Part model, mm, in its own coordinate system. A direction names the side the tool comes from. Give positions to 0.01 mm unless a question says otherwise; leave off trailing zeros. Order: outer loops, then holes, each group sorted by start corner. A loop starts at its lowest first (then second) coordinate and runs counter-clockwise, first axis right, second up. Notation, with made-up numbers: M 42,81 L 59,81 A18 ccw 59,113 Z; hole C 31,-32.5 d11. An arc over 180 degrees is marked long. One line per question, with ' | ' between items.
```python
from build123d import *

# Parameters (mm, degrees)
SKETCH1_R           = 10.5
BOSS_EXTRUDE1_DEPTH = 35
SKETCH1_3_R         = 3
SKETCH1_3_R_2       = 1.1
BOSS_EXTRUDE2_DEPTH = 4
SKETCH2_R           = 11.5
SKETCH2_R_2         = 10.5
CUT_EXTRUDE1_DEPTH  = 30
SKETCH2_3_R         = 4
SKETCH2_3_R_2       = 1.6
BOSS_EXTRUDE3_DEPTH = 6
FILLET1_R           = 3
SKETCH3_R           = 3
CUT_EXTRUDE2_DEPTH  = 54.516726423


with BuildPart() as part:
    # Sketch1 → Boss-Extrude1 (new body)
    with BuildSketch(Plane.XY):
        with BuildLine():
            ThreePointArc((3, 15), (0, 12), (-3, 15))
            Line((-3, 15), (-3, 19.773719933))
            ThreePointArc((-3, 19.773719933), (-17.320508076, 10), (-18.62454379, -7.288783755))
            Line((-18.62454379, -7.288783755), (-14.490381057, -4.901923789))
            ThreePointArc((-14.490381057, -4.901923789), (-11.490381057, -4.901923789), (-9.990381057, -7.5))
            ThreePointArc((-9.990381057, -7.5), (-10.392304845, -9), (-11.490381057, -10.098076211))
            Line((-11.490381057, -10.098076211), (-15.62454379, -12.484936178))
            ThreePointArc((-15.62454379, -12.484936178), (0, -20), (15.62454379, -12.484936178))
            Line((15.62454379, -12.484936178), (11.490381057, -10.098076211))
            ThreePointArc((11.490381057, -10.098076211), (10.392304845, -6), (14.490381057, -4.901923789))
            Line((14.490381057, -4.901923789), (18.62454379, -7.288783755))
            ThreePointArc((18.62454379, -7.288783755), (19.653127942, -3.708714347), (20, 0))
            ThreePointArc((20, 0), (15.165750888, 13.03840481), (3, 19.773719933))
            Line((3, 19.773719933), (3, 15))
        make_face()
        Circle(SKETCH1_R, mode=Mode.SUBTRACT)
    extrude(amount=BOSS_EXTRUDE1_DEPTH)

    # Sketch1_3 → Boss-Extrude2 (add)
    with BuildSketch(Plane.XY):
        with BuildLine():
            ThreePointArc((15.62454379, -12.484936178), (17.320508076, -10), (18.62454379, -7.288783755))
            Line((18.62454379, -7.288783755), (14.490381057, -4.901923789))
            ThreePointArc((14.490381057, -4.901923789), (15.588457268, -6), (15.990381057, -7.5))
            ThreePointArc((15.990381057, -7.5), (14.490381057, -10.098076211), (11.490381057, -10.098076211))
            Line((11.490381057, -10.098076211), (15.62454379, -12.484936178))
        make_face()
        with Locations((12.990381057, -7.5)):
            Circle(SKETCH1_3_R)
        with Locations((12.990381057, -7.5)):
            Circle(SKETCH1_3_R_2, mode=Mode.SUBTRACT)
        with Locations((-12.990381057, -7.5)):
            Circle(SKETCH1_3_R)
        with Locations((-12.990381057, -7.5)):
            Circle(SKETCH1_3_R_2, mode=Mode.SUBTRACT)
        with BuildLine():
            Line((-14.490381057, -4.901923789), (-18.62454379, -7.288783755))
            ThreePointArc((-18.62454379, -7.288783755), (-17.320508076, -10), (-15.62454379, -12.484936178))
            Line((-15.62454379, -12.484936178), (-11.490381057, -10.098076211))
            ThreePointArc((-11.490381057, -10.098076211), (-15.588457268, -9), (-14.490381057, -4.901923789))
        make_face()
        with BuildLine():
            Line((-3, 19.773719933), (-3, 15))
            ThreePointArc((-3, 15), (0, 18), (3, 15))
            Line((3, 15), (3, 19.773719933))
            ThreePointArc((3, 19.773719933), (0, 20), (-3, 19.773719933))
        make_face()
        with Locations((0, 15)):
            Circle(SKETCH1_3_R)
        with Locations((0, 15)):
            Circle(SKETCH1_3_R_2, mode=Mode.SUBTRACT)
    extrude(amount=BOSS_EXTRUDE2_DEPTH)

    # Sketch2 → Cut-Extrude1 (cut)
    with BuildSketch(Plane.XY.offset(35)):
        Circle(SKETCH2_R)
        Circle(SKETCH2_R_2, mode=Mode.SUBTRACT)
    extrude(amount=-CUT_EXTRUDE1_DEPTH, mode=Mode.SUBTRACT)

    # Sketch2_3 → Boss-Extrude3 (add)
    with BuildSketch(Plane.XY.offset(35)):
        with BuildLine():
            ThreePointArc((-19.595917942, -4), (-20, 0), (-19.595917942, 4))
            Line((-19.595917942, 4), (-31.2, 4))
            ThreePointArc((-31.2, 4), (-28.371572875, 2.828427125), (-27.2, 0))
            ThreePointArc((-27.2, 0), (-28.371572875, -2.828427125), (-31.2, -4))
            Line((-31.2, -4), (-19.595917942, -4))
        make_face()
        with Locations((-31.2, 0)):
            Circle(SKETCH2_3_R)
        with Locations((-31.2, 0)):
            Circle(SKETCH2_3_R_2, mode=Mode.SUBTRACT)
        with BuildLine():
            ThreePointArc((31.2, -4), (27.2, 0), (31.2, 4))
            Line((31.2, 4), (19.595917942, 4))
            ThreePointArc((19.595917942, 4), (19.89872306, 2.01017924), (20, 0))
            ThreePointArc((20, 0), (19.89872306, -2.01017924), (19.595917942, -4))
            Line((19.595917942, -4), (31.2, -4))
        make_face()
        with Locations((31.2, 0)):
            Circle(SKETCH2_3_R)
        with Locations((31.2, 0)):
            Circle(SKETCH2_3_R_2, mode=Mode.SUBTRACT)
    extrude(amount=-BOSS_EXTRUDE3_DEPTH)

    # Fillet1
    fillet1_edges = [part.edges().sort_by_distance(p)[0] for p in [
        (-20, 0, 29),
        (19.595917942, -4, 32),
        (19.595917942, 4, 32),
        (20, 0, 29),
        (-19.595917942, 4, 32),
        (-19.595917942, -4, 32),
    ]]
    fillet(fillet1_edges, radius=FILLET1_R)

    # Sketch3 → Cut-Extrude2 (cut, through all)
    with BuildSketch(Plane(origin=(0, 0, 0), x_dir=(1, 0, 0), z_dir=(0, 1, 0))):
        with Locations(Location((0, -13.5, 0), (0, 0, 270))):
            Circle(SKETCH3_R)
    extrude(amount=-CUT_EXTRUDE2_DEPTH, mode=Mode.SUBTRACT)


solid = part.part
```
1. Slice it at A-A on x = 0. Give the cut face in (y, z), then the cut area to 3 significant figures.
Worked out:
outline: M -20,0 L -10.5,0 L -10.5,5 L -11.5,5 L -11.5,10.5 L -20,10.5 Z; M -20,16.5 L -11.5,16.5 L -11.5,35 L -20,35 Z; M 10.5,0 L 13.9,0 L 13.9,4 L 12,4 L 12,35 L 11.5,35 L 11.5,5 L 10.5,5 Z; M 16.1,0 L 20,0 L 20,4 L 16.1,4 Z | area: 297 mm2
2. Slice it at C-C on z = 20. Give the cut face in (x, y), then the cut area to 3 significant figures.
Worked out:
outline: M -18.62,-7.29 L -14.49,-4.9 A3 cw -11.49,-10.1 L -15.62,-12.48 A20 ccw 15.62,-12.48 L 11.49,-10.1 A3 cw 14.49,-4.9 L 18.62,-7.29 A20 ccw 3,19.77 L 3,15 A3 cw -3,15 L -3,19.77 A20 ccw Z; hole C 0,0 d23 | area: 710 mm2
3. Slice it at D-D on z = 27. Give the cut face in (x, y).
Worked out:
outline: M -19.48,-5.24 A3 cw -19.05,-6.09 A20 ccw -18.62,-7.29 L -14.49,-4.9 A3 cw -11.49,-10.1 L -15.62,-12.48 A20 ccw 15.62,-12.48 L 11.49,-10.1 A3 cw 14.49,-4.9 L 18.62,-7.29 A20 ccw 19.05,-6.09 A3 cw 19.48,-5.24 A20.17 ccw 19.48,5.24 A3 cw 19.05,6.09 A20 ccw 3,19.77 L 3,15 A3 cw -3,15 L -3,19.77 A20 ccw -19.05,6.09 A3 cw -19.48,5.24 A20.17 ccw Z; hole C 0,0 d23
4. Drop flat-ended pins along their axis: pin 1 (5 mm diameter, centred on x = -28.5, z = 32.5, fed in from +Y); pin 2 (4 mm diameter, centred on x = -27.5, y = 1.5, fed in from -Z); pin 3 (2.5 mm diameter, centred on x = 14.5, y = -8.5, fed in from +Z). Give the stop position or say it passes through.
Worked out:
pin 1: stops at y = 4 | pin 2: stops at z = 29 | pin 3: stops at z = 4
5. Slice it at B-B on z = 31.5. Give the cut face in (x, y).
Worked out:
outline: M -31.2,-4 L -21.91,-4 A3 cw -19.05,-6.09 A20 ccw -18.62,-7.29 L -14.49,-4.9 A3 cw -11.49,-10.1 L -15.62,-12.48 A20 ccw 15.62,-12.48 L 11.49,-10.1 A3 cw 14.49,-4.9 L 18.62,-7.29 A20 ccw 19.05,-6.09 A3 cw 21.91,-4 L 31.2,-4 A4 ccw 31.2,4 L 21.91,4 A3 cw 19.05,6.09 A20 ccw 3,19.77 L 3,15 A3 cw -3,15 L -3,19.77 A20 ccw -19.05,6.09 A3 cw -21.91,4 L -31.2,4 A4 ccw Z; hole C -31.2,0 d3.2; hole C 0,0 d23; hole C 31.2,0 d3.2
6. Mould opens along Z. For faces 5 (the flat face through (-14.4, -8.4, 4)), 6 (the cylindrical face through (0.1, -15.5, 10.5)), 7 (the cylindrical face through (20.161, -4.562, 31.437)) say: released by +Z, released by -Z, zero draft, split by the parting line, or undercut.
Worked out:
face 5: released by +Z | face 6: undercut | face 7: zero draft
7. Tool access for faces 1 (the flat face through (13.59, -11.31, 19.28)), 2 (the flat face through (-13.529, -11.275, 19.283)), 3 (the flat face through (-3, 17, 19)), 4 (the flat face through (14.2, -8.4, 4)): list every direction of +Z, -Z, +X, -X, +Y, -Y with a clear straight run to the whole face (end or side of a thin tool).
Worked out:
face 1: +Z, +X | face 2: +Z, -X | face 3: +Z, +Y | face 4: +Z
8. Probe L1, parallel to Y at x = 0, z = 2.6; L2, parallel to Y at x = 31, z = 31; L3, parallel to X at y = -7, z = 1 (3 decimals). List the from-to ranges inside material, lowest first. Write a range as from..to.
Worked out:
L1: y = -20..-10.5, 10.5..13.9, 16.1..20 | L2: y = -4..-1.59, 1.59..4 | L3: x = -18.735..-13.97, -12.011..-7.826, 7.826..12.011, 13.97..18.735
